from build123d import *

# Parameters (mm, degrees)
SCHIZZO1_R                   = 2.5
ESTRUSIONE_ESTRUSIONE3_DEPTH = 3


with BuildPart() as part:
    # Schizzo1 → Estrusione-Estrusione3 (new body)
    with BuildSketch(Plane.XY):
        with BuildLine():
            Line((-10, 75), (0, 75))
            Line((0, 75), (0, 66.92820323))
            ThreePointArc((0, 66.92820323), (-4, 60), (0, 53.07179677))
            Line((0, 53.07179677), (0, 0))
            Line((0, 0), (-10, 0))
            Line((-10, 0), (-10, 49.607695155))
            ThreePointArc((-10, 49.607695155), (-16, 60), (-10, 70.392304845))
            Line((-10, 70.392304845), (-10, 75))
        make_face()
        with Locations((-5, 70)):
            Circle(SCHIZZO1_R, mode=Mode.SUBTRACT)
        with Locations((-5, 5)):
            Circle(SCHIZZO1_R, mode=Mode.SUBTRACT)
    extrude(amount=ESTRUSIONE_ESTRUSIONE3_DEPTH)


solid = part.part
Check sheet for the modelled part. Datum: model origin and axes. Units: mm. A direction names the side the tool comes from. Coordinates: 2 decimals unless noted, no trailing zeros. Write each loop counter-clockwise with the first axis right and the second up, starting at its lowest first coordinate (ties: lowest second). Pieces come first, ordered by that corner, then holes. Notation, with made-up numbers: M -16.5,19 L 25.5,19 A22 ccw 25.5,47 Z; hole C -2.5,-38.5 d8. An arc over 180 degrees is marked long. Answer as CSV lines item,"result".
Q1. Go/stop test with flat-tipped pins: pin 1 (4 mm diameter, centred on x = -13.5, y = 36, fed in from +Z); pin 2 (1 mm diameter, centred on x = -14, z = 1.5, fed in from -Y). Record where each tip stops, or that it passes through.
Check result:
pin 1,"through"
pin 2,"y = 52.67"
Q2. Set-up check for faces 4 (the face through (-10, 73, 1)), 5 (the face through (-4, 60, 1)), 6 (the face through (-10, 24, 1)): record each of +Z, -Z, +X, -X, +Y, -Y from which the full face is reachable in a straight line by a thin tool's end or side.
Check result:
face 4,"+Z, -Z, -X, +Y"
face 5,"+Z, -Z, +X"
face 6,"+Z, -Z, -X, -Y"
Q3. Cross-section at D-D (x = -15). Record the boundary of the cut face in (y, z).
Check result:
outline,"M 55.2,0 L 64.8,0 L 64.8,3 L 55.2,3 Z"
Q4. Cross-section at C-C (z = 1.35). Record the boundary of the cut face in (x, y), then the cut area to 3 significant figures.
Check result:
outline,"M -10,0 L 0,0 L 0,53.07 A8 cw 0,66.93 L 0,75 L -10,75 L -10,70.39 A12 ccw -10,49.61 Z; hole C -5,5 d5; hole C -5,70 d5"
area,"760 mm^2"
Q5. Cross-section at B-B (x = -5). Record the boundary of the cut face in (y, z), then the cut area to 3 significant figures.
Check result:
outline,"M 0,0 L 2.5,0 L 2.5,3 L 0,3 Z; M 7.5,0 L 67.5,0 L 67.5,3 L 7.5,3 Z; M 72.5,0 L 75,0 L 75,3 L 72.5,3 Z"
area,"195 mm^2"
Q6. Mould release check, pull along X, two halves, no side actions. Record for faces 1 (the face through (-2.615, 5.751, 1.479)), 2 (the face through (-16, 60, 1)), 3 (the face through (-6, 38, 3)): released by +X, released by -X, zero draft, split by the parting line, or undercut.
Check result:
face 1,"undercut"
face 2,"released by -X"
face 3,"zero draft"
Q7. Material ranges on probe 1 along Y at (x, z) = (-5, 1.35); probe 2 along Y at (x, z) = (-6, 0.1); probe 3 along X at (y, z) = (27, 1.1), recorded low to high. Write a range as from..to.
Check result:
probe 1,"0..2.5, 7.5..67.5, 72.5..75"
probe 2,"0..2.71, 7.29..67.71, 72.29..75"
probe 3,"-10..0"
Q8. Cross-section at A-A (y = 5). Record the boundary of the cut face in (x, z), then the cut area to 3 significant figures.
Check result:
outline,"M -10,0 L -7.5,0 L -7.5,3 L -10,3 Z; M -2.5,0 L 0,0 L 0,3 L -2.5,3 Z"
area,"15.0 mm^2"
